The drawing under review shows one solid part. Ordinate dimensions are in mm from its lowest x, y, z. A direction names the side the tool comes from. Give positions to 0.01 mm unless a question says otherwise; leave off trailing zeros. Write each loop counter-clockwise with the first axis right and the second up, starting at its lowest first coordinate (ties: lowest second). Pieces come first, ordered by that corner, then holes.
Q1. We need section B-B (z = 41.5). Write out the cut boundary in (x, y), then the cut area to 3 significant figures.
Q2. We need section D-D (y = 11). Write out the cut boundary in (x, z).
Q3. For line 1 (Y direction, x = 44, z = 19.5); line 2 (Z direction, x = 46.5, y = 19); line 3 (X direction, y = 96, z = 49) (1 decimal), list the stretches that pass through material, from the lowest coordinate up.
Q4. We need section A-A (z = 12). Write out the cut boundary in (x, y).
Q5. We need section C-C (x = 37). Write out the cut boundary in (y, z), then the cut area to 3 significant figures.
Q6. Insertion check: P1, Ø10, axis at x = 7, y = 53.5, coming from the -Z side; P2, Ø5, axis at x = 20.5, y = 60.5, coming from the +Z side. Each pin has a flat end and moves straight along its axis. Give the tip position at first contact, or say it passes through.
Q7. Mouldability with a two-part tool opening along Y and no side actions: class the marked faces 3, 4 and 5 as released by +Y, released by -Y, zero draft, split by the parting line, or undercut.
Q8. Machinability: for the marked faces 1 and 2, which of the approach directions +Z, -Z, +X, -X, +Y, -Y give a long, thin tool a straight path to every point of the face, cutting with its end or side? Answer none if there is none.
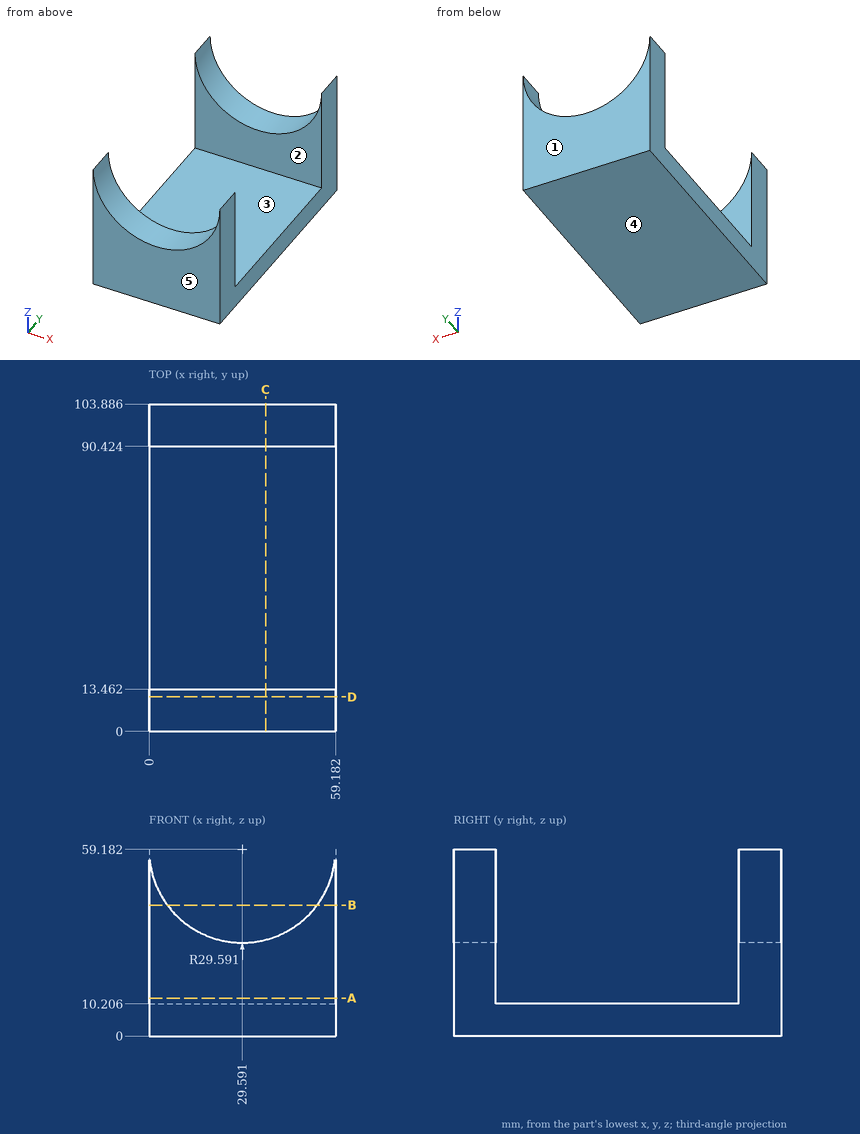
Computed:
1. outline: (0, 0) - (5.86, 0) - (5.86, 13.46) - (0, 13.46) - close; (0, 90.42) - (5.86, 90.42) - (5.86, 103.89) - (0, 103.89) - close; (53.32, 0) - (59.18, 0) - (59.18, 13.46) - (53.32, 13.46) - close; (53.32, 90.42) - (59.18, 90.42) - (59.18, 103.89) - (53.32, 103.89) - close
1. area: 316 mm2
2. outline: (0, 0) - (59.18, 0) - (59.18, 59.18) arc R29.59 cw to (0, 59.18) - close
3. line 1: y = 0 to 13.46, 90.42 to 103.89
3. line 2: z = 0 to 10.21
3. line 3: x = 0 to 1.8, 57.4 to 59.2
4. outline: (0, 0) - (59.18, 0) - (59.18, 13.46) - (0, 13.46) - close; (0, 90.42) - (59.18, 90.42) - (59.18, 103.89) - (0, 103.89) - close
5. outline: (0, 0) - (103.89, 0) - (103.89, 30.53) - (90.42, 30.53) - (90.42, 10.21) - (13.46, 10.21) - (13.46, 30.53) - (0, 30.53) - close
5. area: 1,610 mm2
6. P1: stops at z = 0
6. P2: stops at z = 10.21
7. face 3: undercut
7. face 4: zero draft
7. face 5: released by -Y
8. face 1: +Z, -Z, +X, -X, +Y
8. face 2: +Z, +X, -X
